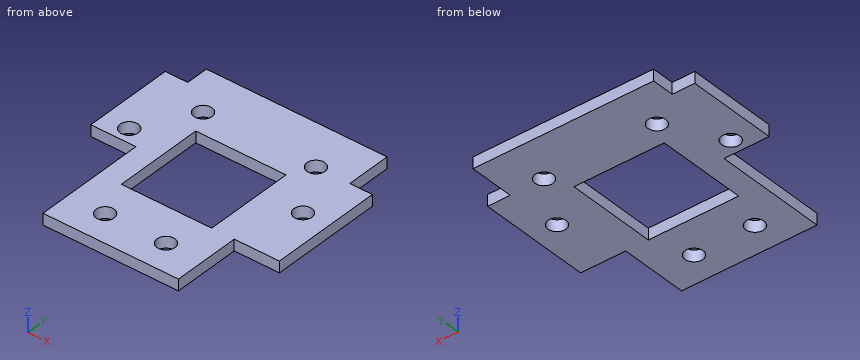
```python
from build123d import *

# Parameters (mm, degrees)
F0_R     = 4
F0_W     = 40
F0_H     = 40
F1_DEPTH = 5


with BuildPart() as f1:
    # F0 (on Top) → F1 (new body)
    with BuildSketch(Plane.XY):
        Polygon((40, 50), (-40, 50), (-40, 40), (-50, 40), (-50, 0), (-30, 0), (-30, -50), (30, -50), (30, -20), (50, -20), (50, 30), (40, 30), align=None)
        with Locations((-13.480762, -36.650635)):
            Circle(F0_R, mode=Mode.SUBTRACT)
        with Locations((13.480762, -36.650635)):
            Circle(F0_R, mode=Mode.SUBTRACT)
        with Locations((-38.480762, 6.650635)):
            Circle(F0_R, mode=Mode.SUBTRACT)
        with Locations((-25, 30)):
            Circle(F0_R, mode=Mode.SUBTRACT)
        Rectangle(F0_W, F0_H, mode=Mode.SUBTRACT)
        with Locations((38.480762, 6.650635)):
            Circle(F0_R, mode=Mode.SUBTRACT)
        with Locations((25, 30)):
            Circle(F0_R, mode=Mode.SUBTRACT)
    extrude(amount=F1_DEPTH)


solid = f1.part
```
Build history of the part. All positions in model axes, mm. Give positions to 0.01 mm unless a question says otherwise; leave off trailing zeros. Loops run counter-clockwise (first coordinate to the right, second up) from the corner with the lowest first, then second, coordinate; pieces in that order, holes last.
1) Band-saw the part on B-B on y = -10.5. List the corners of the cut face in (x, z), then the cut area to 3 significant figures.
Values follow:
outline: (-30, 0) - (-20, 0) - (-20, 5) - (-30, 5) - close; (20, 0) - (50, 0) - (50, 5) - (20, 5) - close
area: 200 mm2
2) Band-saw the part on A-A on x = 7. List the corners of the cut face in (y, z).
Values follow:
outline: (-50, 0) - (-20, 0) - (-20, 5) - (-50, 5) - close; (20, 0) - (50, 0) - (50, 5) - (20, 5) - close
3) Drop flat-ended pins along their axis: P1, Ø2.5, axis at x = 44, z = 2, coming from the +Y side; P2, Ø1.5, axis at x = -41.5, z = 3, coming from the -Y side. Give the stop position or say it passes through.
Values follow:
P1: stops at y = 30
P2: stops at y = 0
4) Band-saw the part on D-D on y = -22. List the corners of the cut face in (x, z), then the cut area to 3 significant figures.
Values follow:
outline: (-30, 0) - (30, 0) - (30, 5) - (-30, 5) - close
area: 300 mm2
5) Probe line 1 along X through (y, z) = (-0.5, 3.75); line 2 along Y through (x, z) = (13.5, 4.2); line 3 along X through (y, z) = (10, 1.55). List the from-to ranges inside material, lowest first.
Values follow:
line 1: x = -30 to -20, 20 to 50
line 2: y = -50 to -40.65, -32.65 to -20, 20 to 50
line 3: x = -50 to -40.67, -36.29 to -20, 20 to 36.29, 40.67 to 50
6) Band-saw the part on C-C on z = 3.6. List the corners of the cut face in (x, y), then the cut area to 3 significant figures.
Values follow:
outline: (-50, 0) - (-30, 0) - (-30, -50) - (30, -50) - (30, -20) - (50, -20) - (50, 30) - (40, 30) - (40, 50) - (-40, 50) - (-40, 40) - (-50, 40) - close; hole circle Ø8 at (-38.48, 6.65); hole circle Ø8 at (-25, 30); hole (-20, -20) - (20, -20) - (20, 20) - (-20, 20) - close; hole circle Ø8 at (-13.48, -36.65); hole circle Ø8 at (13.48, -36.65); hole circle Ø8 at (25, 30); hole circle Ø8 at (38.48, 6.65)
area: 6,200 mm2
